from build123d import *

# Parameters (mm, degrees)
F1_DEPTH = 80
F2_W     = 170
F2_H     = 27.5
F3_DEPTH = 30
F6_DEPTH = 65
F8_R     = 15
F9_DEPTH = 20


with BuildPart() as f1:
    # F0 (on Front) → F1 (new body)
    with BuildSketch(Plane.XZ):
        with BuildLine():
            ThreePointArc((110, 2.5), (102.6776695297, 20.1776695297), (85, 27.5))
            Line((85, 27.5), (-85, 27.5))
            ThreePointArc((-85, 27.5), (-102.6776695297, 20.1776695297), (-110, 2.5))
            Line((-110, 2.5), (-110, -27.5))
            Line((-110, -27.5), (110, -27.5))
            Line((110, -27.5), (110, 2.5))
        make_face()
    extrude(amount=F1_DEPTH)

    # F2 (on face) → F3 (cut)
    with BuildSketch(Plane.XZ.offset(80)):
        with Locations((0, -13.75)):
            Rectangle(F2_W, F2_H)
    extrude(amount=-F3_DEPTH, mode=Mode.SUBTRACT)

    # F5 (on offset) → F6 (join)
    with BuildSketch(Plane.XZ.offset(65)):
        with BuildLine():
            Line((-46.5551204979, 112.5), (-63.5551204979, 112.5))
            Line((-63.5551204979, 112.5), (-63.5551204979, 27.5))
            Line((-63.5551204979, 27.5), (66.4448795021, 27.5))
            Line((66.4448795021, 27.5), (66.4448795021, 112.5))
            Line((66.4448795021, 112.5), (49.4448795021, 112.5))
            ThreePointArc((49.4448795021, 112.5), (1.4448795021, 64.5), (-46.5551204979, 112.5))
        make_face()
    extrude(amount=-F6_DEPTH)

    # F8 (on offset) → F9 (join)
    with BuildSketch(Plane.XZ):
        with BuildLine():
            Line((100, 107.5), (66.4448795021, 107.5))
            Line((66.4448795021, 107.5), (66.4448795021, 27.5))
            Line((66.4448795021, 27.5), (85, 27.5))
            ThreePointArc((85, 27.5), (102.6776695297, 20.1776695297), (110, 2.5))
            Line((110, 2.5), (110, -27.5))
            Line((110, -27.5), (145, -27.5))
            Line((145, -27.5), (145, 62.5))
            ThreePointArc((145, 62.5), (131.8198051534, 94.3198051534), (100, 107.5))
        make_face()
        with Locations((105.722439751, 80.8619317412)):
            Circle(F8_R, mode=Mode.SUBTRACT)
        with BuildLine():
            ThreePointArc((-100, 107.5), (-131.8198051534, 94.3198051534), (-145, 62.5))
            Line((-145, 62.5), (-145, -27.5))
            Line((-145, -27.5), (-110, -27.5))
            Line((-110, -27.5), (-110, 2.5))
            ThreePointArc((-110, 2.5), (-102.6776695297, 20.1776695297), (-85, 27.5))
            Line((-85, 27.5), (-63.5551204979, 27.5))
            Line((-63.5551204979, 27.5), (-63.5551204979, 107.5))
            Line((-63.5551204979, 107.5), (-100, 107.5))
        make_face()
        with Locations((-105.722439751, 80.8619317412)):
            Circle(F8_R, mode=Mode.SUBTRACT)
    extrude(amount=F9_DEPTH)


solid = f1.part
Check sheet for the modelled part. Datum: model origin and axes. Units: mm. A direction names the side the tool comes from. Give positions to 0.01 mm unless a question says otherwise; leave off trailing zeros. Write each loop counter-clockwise with the first axis right and the second up, starting at its lowest first coordinate (ties: lowest second). Pieces come first, ordered by that corner, then holes. Notation, with made-up numbers: (40, 40) -> (95, 40) arc R9 cw to (95, 50) -> close; hole circle Ø2 at (83.5, 89.25). An arc over 180 degrees is marked (long way). Use one line per item in the form item = value. Start each with the question number.
1. Section check D-D (z = 71). Record the cut outline in (x, y).
2. Access from +Z, -Z, +X, -X, +Y, -Y to the whole of each face (thin tool, end or side, straight path). Record for faces 4 (the flat face through (1, -65, 61)), 5 (the flat face through (-82, -10, 107.5)), 6 (the flat face through (114, -20, 41)), 7 (the cylindrical face through (-102.482, -49.58, 20.371)), 8 (the flat face through (-110, -50, -12)).
3. Section check C-C (x = 80.5). Record the cut outline in (y, z), and give its area (4 significant figures).
4. Thickness scan on line 1 along X through (y, z) = (-13, 87.5); line 2 along Y through (x, z) = (-15.5, 44); line 3 along X through (y, z) = (-35, 57). Record the ranges inside material, lowest first. Write a range as from..to.
5. Section check B-B (y = -54.5). Record the cut outline in (x, z), and give its area (3 significant figures).
6. Go/stop test with flat-tipped pins: P1, Ø8, axis at y = -71, z = -11.5, coming from the -X side; P2, Ø1.5, axis at x = 111.5, z = 68, coming from the -Y side; P3, Ø4, axis at x = -76.5, y = -58, coming from the -Z side; P4, Ø15, axis at y = -42.5, z = -14, coming from the +X side. Record where each tip stops, or that it passes through.
7. Mould release check, pull along X, two halves, no side actions. Record for faces 1 (the cylindrical face through (-131.468, -9.86, 94.668)), 2 (the flat face through (83, -10, 107.5)), 3 (the flat face through (-1, -50, -14)): pulls with the +X half, pulls with the -X half, needs draft (parallel to the pull), parting line crosses it, or undercut.
8. Section check A-A (z = -16.5). Record the cut outline in (x, y), and give its area (3 significant figures).
Conclusion:
q1.outline = (-144.19, -20) -> (-117.02, -20) -> (-117.02, 0) -> (-144.19, 0) -> close; (-94.42, -20) -> (-63.56, -20) -> (-63.56, -65) -> (-22.67, -65) -> (-22.67, 0) -> (-94.42, 0) -> close; (25.56, -65) -> (66.44, -65) -> (66.44, -20) -> (94.42, -20) -> (94.42, 0) -> (25.56, 0) -> close; (117.02, -20) -> (144.19, -20) -> (144.19, 0) -> (117.02, 0) -> close
q2.face_4 = +Z, +X, -X, -Y
q2.face_5 = +Z, -X, +Y, -Y
q2.face_6 = +Z, +X, -Y
q2.face_7 = +Z, -X, -Y
q2.face_8 = +Z, -Z, -X, -Y
q3.outline = (-80, 0) -> (-50, 0) -> (-50, -27.5) -> (0, -27.5) -> (0, 107.5) -> (-20, 107.5) -> (-20, 27.5) -> (-80, 27.5) -> close
q3.area = 5,175 mm²
q4.line_1 = -137.42..-119.17, -92.27..-39.53, 42.42..92.27, 119.17..137.42
q4.line_2 = -65..0
q4.line_3 = -63.56..66.44
q5.outline = (-110, -27.5) -> (-85, -27.5) -> (-85, 0) -> (85, 0) -> (85, -27.5) -> (110, -27.5) -> (110, 2.5) arc R25 ccw to (85, 27.5) -> (66.44, 27.5) -> (66.44, 112.5) -> (49.44, 112.5) arc R48 cw to (-46.56, 112.5) -> (-63.56, 112.5) -> (-63.56, 27.5) -> (-85, 27.5) arc R25 ccw to (-110, 2.5) -> close
q5.area = 14,600 mm²
q6.P1 = -110
q6.P2 = through
q6.P3 = 0
q6.P4 = 110
q7.face_1 = pulls with the -X half
q7.face_2 = needs draft
q7.face_3 = undercut
q8.outline = (-145, -20) -> (-110, -20) -> (-110, -80) -> (-85, -80) -> (-85, -50) -> (85, -50) -> (85, -80) -> (110, -80) -> (110, -20) -> (145, -20) -> (145, 0) -> (-145, 0) -> close
q8.area = 13,900 mm²
